Autodesk Fusion 360 part; units mm, degrees
sketch "Sketch1" plane through (0, 0, 0) normal (0, 1, 0) x (1, 0, 0)
  line L0 (-4, 40) -> (4, 40)
  line L1 (4, 40) -> (4, 0)
  line L2 (4, 0) -> (-4, 0)
  line L3 (-4, 0) -> (-4, 40)
  point P0 (0, 4)
  point P1 (0, 14)
  dimension "d1" = 8
  dimension "d2" = 40
  dimension "d3" = 4
  dimension "d4" = 10
extrude "Extrude1" add sketch "Sketch1" along normal blind 2
hole "Hole1" at (0, 0, -4) direction (0, 1, 0) diameter 5.5 depth 16 tip angle 118
hole "Hole2" at (0, 0, -14) direction (0, 1, 0) diameter 1.623 depth 16 tip angle 118
pattern_linear "R-Pattern1" count 5 spacing 5 along (0, 0, -1) of "Hole2"
chamfer "Chamfer1" distance 0.5 angle 45 4 edges at (4, 1, 0) (-4, 1, 0) (4, 1, -40) (-4, 1, -40)
Read the model definition and answer for the solid it produces. Units are mm, in the model's axes. Round coordinates to 2 decimals unless told otherwise and drop trailing zeros. Loops run counter-clockwise (first coordinate to the right, second up) from the corner with the lowest first, then second, coordinate; pieces in that order, holes last. Notation, with made-up numbers: (11.25, 66) -> (54.25, 66) arc R23 cw to (54.25, 98) -> close; hole circle Ø8 at (74, 34.25). An arc over 180 degrees is marked (long way). One line per item, written item: value.
1) A flat-ended cylindrical pin translates along its axis: P1, Ø1.3, axis at x = 0, z = -29, coming from the -Y side. Find the tip coordinate at first contact, or state that the pin passes through.
Answer list:
P1: passes through
2) A cutting plane is placed at B-B (z = -24). Determine the outline of the cut face in (x, y), and give its area (3 significant figures).
Answer list:
outline: (-4, 0) -> (-0.81, 0) -> (-0.81, 2) -> (-4, 2) -> close; (0.81, 0) -> (4, 0) -> (4, 2) -> (0.81, 2) -> close
area: 12.8 mm²
3) A cutting plane is placed at D-D (x = -1.75). Determine the outline of the cut face in (y, z).
Answer list:
outline: (0, -40) -> (2, -40) -> (2, -6.12) -> (0, -6.12) -> close; (0, -1.88) -> (2, -1.88) -> (2, 0) -> (0, 0) -> close
4) The mould has two halves that part along X. Classify faces 1 (the face through (0.31, 1.01, -34.75)), 2 (the face through (-4, 1, -20)), 3 (the face through (0, 1, 0)): pulls with the +X half, pulls with the -X half, needs draft (parallel to the pull), parting line crosses it, or undercut.
Answer list:
face 1: undercut
face 2: pulls with the -X half
face 3: needs draft
5) Consider L1, parallel to X at y = 1.5, z = -19; L2, parallel to Z at x = 2.5, y = 1.1; L3, parallel to Z at x = -1.5, y = 0.75. Determine where each line is inside the solid, lowest interval first. Write a range as [from, to].
Answer list:
L1: x = [-4, -0.81], [0.81, 4]
L2: z = [-40, -5.15], [-2.85, 0]
L3: z = [-40, -6.3], [-1.7, 0]
6) A cutting plane is placed at A-A (x = 0). Determine the outline of the cut face in (y, z).
Answer list:
outline: (0, -40) -> (2, -40) -> (2, -34.81) -> (0, -34.81) -> close; (0, -33.19) -> (2, -33.19) -> (2, -29.81) -> (0, -29.81) -> close; (0, -28.19) -> (2, -28.19) -> (2, -24.81) -> (0, -24.81) -> close; (0, -23.19) -> (2, -23.19) -> (2, -19.81) -> (0, -19.81) -> close; (0, -18.19) -> (2, -18.19) -> (2, -14.81) -> (0, -14.81) -> close; (0, -13.19) -> (2, -13.19) -> (2, -6.75) -> (0, -6.75) -> close; (0, -1.25) -> (2, -1.25) -> (2, 0) -> (0, 0) -> close
7) A cutting plane is placed at C-C (y = 1.6). Determine the outline of the cut face in (x, z).
Answer list:
outline: (-4, -39.5) -> (-3.5, -40) -> (3.5, -40) -> (4, -39.5) -> (4, -0.5) -> (3.5, 0) -> (-3.5, 0) -> (-4, -0.5) -> close; hole circle Ø5.5 at (0, -4); hole circle Ø1.62 at (0, -34); hole circle Ø1.62 at (0, -29); hole circle Ø1.62 at (0, -24); hole circle Ø1.62 at (0, -19); hole circle Ø1.62 at (0, -14)
